Source: three-view drawing plus pictorial views. Frame: mm from the lowest corner of the part. A direction names the side the tool comes from. Give positions to 0.01 mm unless a question says otherwise; leave off trailing zeros. Write each loop counter-clockwise with the first axis right and the second up, starting at its lowest first coordinate (ties: lowest second). Pieces come first, ordered by that corner, then holes. Notation, with made-up numbers: M 24.25,54.5 L 44.25,54.5 A14 cw 44.25,76.5 Z; hole C -22,-16 d4. An arc over 180 degrees is marked long. One line per question, with ' | ' between items.
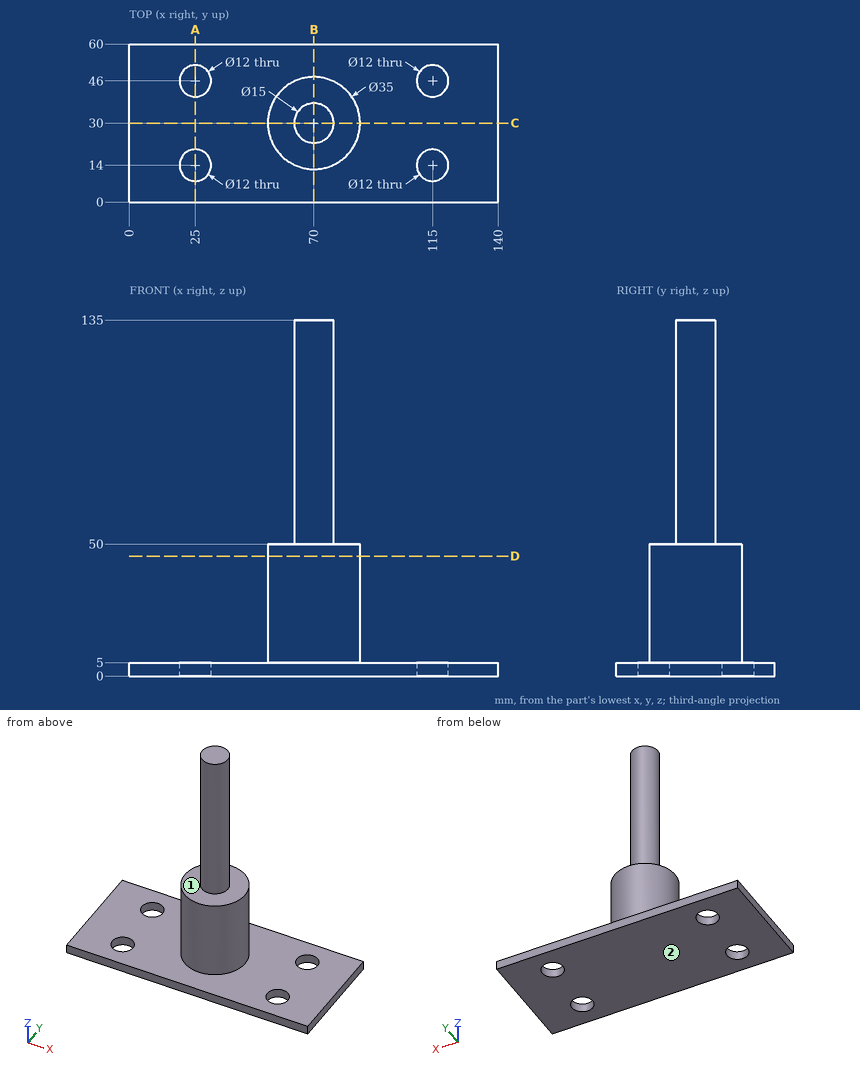
(1) Set-up query: the marked faces 1 and 2. Return all of +Z, -Z, +X, -X, +Y, -Y with unobstructed straight access to the full face (end or side cutting, diameter ignored); none if empty.
Working result:
face 1: +Z | face 2: -Z, +X, -X, +Y, -Y
(2) Cut plane D-D, the plane z = 45.5. Return loops of the section in (x, y), then the cut area to 3 significant figures.
Working result:
outline: C 70,30 d35 | area: 962 mm^2
(3) Cut plane A-A, the plane x = 25. Return loops of the section in (y, z).
Working result:
outline: M 0,0 L 8,0 L 8,5 L 0,5 Z; M 20,0 L 40,0 L 40,5 L 20,5 Z; M 52,0 L 60,0 L 60,5 L 52,5 Z
(4) Cut plane C-C, the plane y = 30. Return loops of the section in (x, z).
Working result:
outline: M 0,0 L 140,0 L 140,5 L 87.5,5 L 87.5,50 L 77.5,50 L 77.5,135 L 62.5,135 L 62.5,50 L 52.5,50 L 52.5,5 L 0,5 Z
(5) Material intervals for L1, parallel to Y at x = 25, z = 2.7; L2, parallel to Z at x = 91, y = 42; L3, parallel to Z at x = 64.5, y = 20, sorted ascending. Write a range as [from, to].
Working result:
L1: y = [0, 8], [20, 40], [52, 60] | L2: z = [0, 5] | L3: z = [0, 50]
(6) First-contact query: P1, Ø6, axis at x = 92.5, y = 31, coming from the +Z side; P2, Ø7, axis at x = 115, y = 46, coming from the +Z side; P3, Ø2, axis at x = 88, y = 32.5, coming from the -Z side. Flat tips, straight axial feed; report the tip coordinate or a pass-through.
Working result:
P1: stops at z = 5 | P2: passes through | P3: stops at z = 0
(7) Cut plane B-B, the plane x = 70. Return loops of the section in (y, z), then the cut area to 3 significant figures.
Working result:
outline: M 0,0 L 60,0 L 60,5 L 47.5,5 L 47.5,50 L 37.5,50 L 37.5,135 L 22.5,135 L 22.5,50 L 12.5,50 L 12.5,5 L 0,5 Z | area: 3,150 mm^2
